from build123d import *

# Parameters (mm, degrees)
F1_DEPTH = 6.35


with BuildPart() as f1:
    # F0 (on Top) → F1 (new body)
    with BuildSketch(Plane.XY):
        with BuildLine():
            Line((0, -6.279444), (0, 0))
            Line((0, 0), (0, 6.279444))
            Line((0, 6.279444), (-25.4, 6.279444))
            ThreePointArc((-25.4, 6.279444), (-33.943051, 9.557721), (-38.1, 17.709444))
            Line((-38.1, 17.709444), (-50.8, 17.709444))
            Line((-50.8, 17.709444), (-50.8, -20.390556))
            Line((-50.8, -20.390556), (-38.1, -20.390556))
            ThreePointArc((-38.1, -20.390556), (-34.892279, -10.506949), (-25.4, -6.279444))
            Line((-25.4, -6.279444), (0, -6.279444))
        make_face()
        with BuildLine():
            Line((0, 6.279444), (0, 0))
            Line((0, 0), (0, -6.279444))
            Line((0, -6.279444), (25.4, -6.279444))
            ThreePointArc((25.4, -6.279444), (34.892279, -10.506949), (38.1, -20.390556))
            Line((38.1, -20.390556), (50.8, -20.390556))
            Line((50.8, -20.390556), (50.8, 17.709444))
            Line((50.8, 17.709444), (38.1, 17.709444))
            ThreePointArc((38.1, 17.709444), (33.943051, 9.557721), (25.4, 6.279444))
            Line((25.4, 6.279444), (0, 6.279444))
        make_face()
    extrude(amount=F1_DEPTH)


solid = f1.part
Can you work these out from the model? Positions are in its coordinate system, mm. A direction names the side the tool comes from. Give positions to 0.01 mm unless a question says otherwise; leave off trailing zeros. Loops run counter-clockwise (first coordinate to the right, second up) from the corner with the lowest first, then second, coordinate; pieces in that order, holes last. Notation, with made-up numbers: M -24.5,14 L -17.5,14 A20 ccw -17.5,48 Z; hole C 52.25,60 d3. An arc over 180 degrees is marked long. One line per item, written item: value.
1) Thinking about a two-plate mould opening in X: for faces 1 (the face through (-1, -1, 0)), 2 (the face through (50.8, -2, 3)), 3 (the face through (34.04, 9.646, 3.131)), which applies, +X half, -X half, draft (parallel to the pull), parting line (faces both ways), or undercut?
Geometry check:
face 1: draft
face 2: +X half
face 3: undercut
2) Imagine slicing it at B-B on y = 9.5. Write out the boundary of the cut face in (x, z), and give its area (3 significant figures).
Geometry check:
outline: M -50.8,0 L -33.88,0 L -33.88,6.35 L -50.8,6.35 Z; M 33.88,0 L 50.8,0 L 50.8,6.35 L 33.88,6.35 Z
area: 215 mm²
3) On a 3-axis mill with a long thin cutter (end or side, diameter ignored), from which of +Z, -Z, +X, -X, +Y, -Y can I reach the whole of each face in a straight line? I mean faces 4 (the face through (-45, -20.391, 3)), 5 (the face through (0, 6.279, 3)), 6 (the face through (0, -6.279, 3)). Say none if no direction works.
Geometry check:
face 4: +Z, -Z, +X, -X, -Y
face 5: +Z, -Z, +Y
face 6: +Z, -Z, -Y
4) I'm going to push flat-ended pins straight in: pin 1 (2 mm diameter, centred on x = -18, z = 2, fed in from -Y); pin 2 (3 mm diameter, centred on x = -12, z = 3, fed in from +Y). Where does each tip first touch, or does it pass through?
Geometry check:
pin 1: stops at y = -6.28
pin 2: stops at y = 6.28
5) Imagine slicing it at D-D on x = -8. Write out the boundary of the cut face in (y, z).
Geometry check:
outline: M -6.28,0 L 6.28,0 L 6.28,6.35 L -6.28,6.35 Z
6) Please list where these lines run through material, in increasing order: line 1 (Y direction, x = -12, z = 2.75); line 2 (X direction, y = 12, z = 4); line 3 (X direction, y = -17, z = 3.75).
Geometry check:
line 1: y = -6.28 to 6.28
line 2: x = -50.8 to -36.05, 36.05 to 50.8
line 3: x = -50.8 to -38, 38 to 50.8
7) Imagine slicing it at C-C on y = 15. Write out the boundary of the cut face in (x, z).
Geometry check:
outline: M -50.8,0 L -37.51,0 L -37.51,6.35 L -50.8,6.35 Z; M 37.51,0 L 50.8,0 L 50.8,6.35 L 37.51,6.35 Z
8) Imagine slicing it at A-A on z = 3. Write out the boundary of the cut face in (x, y), and give its area (3 significant figures).
Geometry check:
outline: M -50.8,-20.39 L -38.1,-20.39 A12.77 cw -25.4,-6.28 L 25.4,-6.28 A12.77 cw 38.1,-20.39 L 50.8,-20.39 L 50.8,17.71 L 38.1,17.71 A12.77 cw 25.4,6.28 L -25.4,6.28 A12.77 cw -38.1,17.71 L -50.8,17.71 Z
area: 2,060 mm²
